from build123d import *

# Parameters (mm, degrees)
SKETCH_2_R          = 7
EXTRUDE_1_DEPTH     = 10
SKETCH_3_R          = 10
EXTRUDE_2_DEPTH     = 9
SKETCH_4_R          = 3.5
CUT_EXTRUDE_1_DEPTH = 20
CUT_EXTRUDE_START   = -13
SKETCH_5_R          = 5.5
CUT_EXTRUDE_2_DEPTH = 2.5


with BuildPart() as part:
    # Эскиз2 → Бобышка-Вытянуть1 (new body)
    with BuildSketch(Plane.XY):
        Circle(SKETCH_2_R)
    extrude(amount=EXTRUDE_1_DEPTH)

    # Эскиз3 → Бобышка-Вытянуть2 (add)
    with BuildSketch(Plane(origin=(0, 0, 0), x_dir=(-1, 0, 0), z_dir=(0, 0, -1))):
        Circle(SKETCH_3_R)
    extrude(amount=EXTRUDE_2_DEPTH)

    # Эскиз4 → Вырез-Вытянуть1 (cut, through all)
    with BuildSketch(Plane.XY.offset(10)):
        Circle(SKETCH_4_R)
    extrude(amount=-CUT_EXTRUDE_1_DEPTH, mode=Mode.SUBTRACT)

    # Эскиз5 → Вырез-Вытянуть2 (cut)
    with BuildSketch(Plane.XY.offset(10).offset(CUT_EXTRUDE_START)):
        Circle(SKETCH_5_R)
    extrude(amount=-CUT_EXTRUDE_2_DEPTH, mode=Mode.SUBTRACT)


solid = part.part
CAD build for the part. Positions are in the model's coordinates, mm. A direction names the side the tool comes from. Round coordinates to 2 decimals unless told otherwise and drop trailing zeros. Write each loop counter-clockwise with the first axis right and the second up, starting at its lowest first coordinate (ties: lowest second). Pieces come first, ordered by that corner, then holes. Notation, with made-up numbers: M 19,27.5 L 24,27.5 A23 cw 24,36.5 Z; hole C 31.25,-27 d6. An arc over 180 degrees is marked long. Put each result on its own line as item: value. Start each with the question number.
1) Saw through at D-D, the plane x = 4.5. Write the cut outline in (y, z), and give its area (3 significant figures).
2) Saw through at C-C, the plane z = 0.5. Write the cut outline in (x, y).
3) Saw through at A-A, the plane x = 0. Write the cut outline in (y, z).
4) Pull direction Z, two halves, no side cores. Call faces 1 (the cylindrical face through (6.466, -2.681, 4.93)), 2 (the flat face through (7, -2, 0)), 3 (the flat face through (4, 0, -5.5)): pulls with the +Z half, pulls with the -Z half, needs draft (parallel to the pull), parting line crosses it, or undercut.
5) Drill centre lines: probe 1 along Y at (x, z) = (0, 1); probe 2 along Z at (x, y) = (-3, -4); probe 3 along Y at (x, z) = (0, -6.65). Where is each one in solid material? Low to high. Write a range as [from, to].
6) Pin check, flat tips, straight feed: pin 1 Ø2 at (x, z) = (-1, 4.5) entering from +Y; pin 2 Ø6 at (y, z) = (2.5, 3.5) entering from -X; pin 3 Ø8 at (y, z) = (0, 3) entering from +X; pin 4 Ø5 at (y, z) = (6, 8) entering from -X. Stop position of each tip, or through.
7) 3-axis set-ups, long thin cutter, end or side, ignore diameter. For faces 4 (the flat face through (4, 0, -3)), 5 (the cylindrical face through (3.233, -1.341, 3.591)): which of +Z, -Z, +X, -X, +Y, -Y reach the whole face in a straight line?
Resolved:
1. outline: M -8.93,-9 L 8.93,-9 L 8.93,0 L 5.36,0 L 5.36,10 L -5.36,10 L -5.36,0 L -8.93,0 Z; hole M -3.16,-5.5 L 3.16,-5.5 L 3.16,-3 L -3.16,-3 Z
1. area: 252 mm²
2. outline: C 0,0 d14; hole C 0,0 d7
3. outline: M -10,-9 L -3.5,-9 L -3.5,-5.5 L -5.5,-5.5 L -5.5,-3 L -3.5,-3 L -3.5,10 L -7,10 L -7,0 L -10,0 Z; M 3.5,-9 L 10,-9 L 10,0 L 7,0 L 7,10 L 3.5,10 L 3.5,-3 L 5.5,-3 L 5.5,-5.5 L 3.5,-5.5 Z
4. face 1: needs draft
4. face 2: pulls with the +Z half
4. face 3: undercut
5. probe 1: [-7, -3.5], [3.5, 7]
5. probe 2: [-9, -5.5], [-3, 10]
5. probe 3: [-10, -3.5], [3.5, 10]
6. pin 1: y = 7
6. pin 2: x = -7
6. pin 3: x = 10
6. pin 4: x = -6.06
7. face 4: none
7. face 5: +Z, -Z
